Geometry: final body of the model. Coordinates: model frame, mm. Give positions to 0.01 mm unless a question says otherwise; leave off trailing zeros. Loops run counter-clockwise (first coordinate to the right, second up) from the corner with the lowest first, then second, coordinate; pieces in that order, holes last. Notation, with made-up numbers: (1.25, 37) -> (8.25, 37) arc R25 cw to (8.25, 61) -> close; hole circle Ø8 at (64, 53). An arc over 180 degrees is marked (long way). Answer in a Markdown table with one row per item. Add a question column.
1) Section query D-D (z = -40.75). Give the number of separate pieces and of enclosed holes in the cut face, plus the area to 3 significant figures.
2) Section query A-A (x = -1.75). Return the cut outline in (y, z) (3 decimals).
3) Section query B-B (y = 0). Return the cut outline in (x, z) (3 decimals).
4) First-contact query: P1, Ø1.9, axis at x = -19.5, y = 23, coming from the +Z side; P2, Ø2, axis at x = -8.5, z = -38.5, coming from the -Y side; P3, Ø1, axis at y = -26.5, z = -40, coming from the +X side. Flat tips, straight axial feed; report the tip coordinate or a pass-through.
5) Line query: line 1 (Y direction, x = -1.75, z = -40.6); line 2 (Y direction, x = -1.75, z = -37.25) (3 decimals); line 3 (X direction, y = 8, z = -37.2). Output: solid intervals per line, ascending. Write a range as from..to.
6) Section query C-C (x = -11). Return the cut outline in (y, z), plus the area to 3 significant figures.
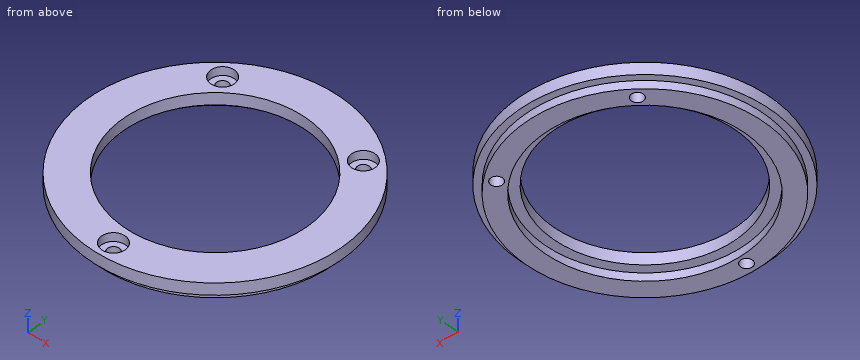
```python
from build123d import *

# Parameters (mm, degrees)
SKETCH018_R     = 32.316823
SKETCH018_R_2   = 27.236823
PAD008_DEPTH    = 2.159
SKETCH019_R     = 34.145623
SKETCH019_R_2   = 24.765
PAD009_DEPTH    = 3.175
SKETCH020_R     = 1.5875
POCKET006_DEPTH = 5.335
SKETCH021_R     = 3.175
POCKET007_DEPTH = 2.286


with BuildPart() as part:
    # Sketch018 (on Face1 of Binder011) → Pad008 (new body)
    with BuildSketch(Plane.XY.offset(-41.598449)):
        with Locations((-1.75, 0)):
            Circle(SKETCH018_R)
        with Locations((-1.75, 0)):
            Circle(SKETCH018_R_2, mode=Mode.SUBTRACT)
    extrude(amount=PAD008_DEPTH)

    # Sketch019 (on Face3 of Pad008) → Pad009 (join)
    with BuildSketch(Plane.XY.offset(-39.439449)):
        with Locations((-1.75, 0)):
            Circle(SKETCH019_R)
        with Locations((-1.75, 0)):
            Circle(SKETCH019_R_2, mode=Mode.SUBTRACT)
    extrude(amount=PAD009_DEPTH)

    # Sketch020 (on Face6 of Pad009) → Pocket006 (cut, through all)
    with BuildSketch(Plane.XY.offset(-36.264449)):
        with Locations((-1.75, -29.645623)):
            Circle(SKETCH020_R)
        with Locations((17.305839, 22.709864)):
            Circle(SKETCH020_R)
        with Locations((-20.805839, 22.709864)):
            Circle(SKETCH020_R)
    extrude(amount=-POCKET006_DEPTH, mode=Mode.SUBTRACT)

    # Sketch021 (on Face9 of Pocket006) → Pocket007 (cut)
    with BuildSketch(Plane.XY.offset(-36.264449)):
        with Locations((-20.805839, 22.709864)):
            Circle(SKETCH021_R)
        with Locations((17.305839, 22.709864)):
            Circle(SKETCH021_R)
        with Locations((-1.75, -29.645623)):
            Circle(SKETCH021_R)
    extrude(amount=-POCKET007_DEPTH, mode=Mode.SUBTRACT)


solid = part.part
```
Evaluation:
| question | item | result |
|---|---|---|
| 1 | separate pieces | 1 |
| 1 | enclosed holes | 4 |
| 1 | area | 927 mm² |
| 2 | outline | (-34.146, -39.439) -> (-32.317, -39.439) -> (-32.317, -41.598) -> (-31.233, -41.598) -> (-31.233, -38.55) -> (-32.821, -38.55) -> (-32.821, -36.264) -> (-34.146, -36.264) -> close; (-28.058, -41.598) -> (-27.237, -41.598) -> (-27.237, -39.439) -> (-24.765, -39.439) -> (-24.765, -36.264) -> (-26.471, -36.264) -> (-26.471, -38.55) -> (-28.058, -38.55) -> close; (24.765, -39.439) -> (27.237, -39.439) -> (27.237, -41.598) -> (32.317, -41.598) -> (32.317, -39.439) -> (34.146, -39.439) -> (34.146, -36.264) -> (24.765, -36.264) -> close |
| 3 | outline | (-35.896, -39.439) -> (-34.067, -39.439) -> (-34.067, -41.598) -> (-28.987, -41.598) -> (-28.987, -39.439) -> (-26.515, -39.439) -> (-26.515, -36.264) -> (-35.896, -36.264) -> close; (23.015, -39.439) -> (25.487, -39.439) -> (25.487, -41.598) -> (30.567, -41.598) -> (30.567, -39.439) -> (32.396, -39.439) -> (32.396, -36.264) -> (23.015, -36.264) -> close |
| 4 | P1 | z = -38.55 |
| 4 | P2 | y = -33.66 |
| 4 | P3 | x = 17.44 |
| 5 | line 1 | -32.32..-31.23, -28.06..-27.24, 27.24..32.32 |
| 5 | line 2 | -34.146..-32.821, -26.471..-24.765, 24.765..34.146 |
| 5 | line 3 | -34.95..-25.19, 21.69..31.45 |
| 6 | outline | (-32.87, -39.44) -> (-30.96, -39.44) -> (-30.96, -41.6) -> (-25.62, -41.6) -> (-25.62, -39.44) -> (-22.97, -39.44) -> (-22.97, -36.26) -> (-32.87, -36.26) -> close; (22.97, -39.44) -> (25.62, -39.44) -> (25.62, -41.6) -> (30.96, -41.6) -> (30.96, -39.44) -> (32.87, -39.44) -> (32.87, -36.26) -> (22.97, -36.26) -> close |
| 6 | area | 85.9 mm² |
